Model file for the job. Use its own axes, mm. Round coordinates to 2 decimals unless told otherwise and drop trailing zeros. Loops run counter-clockwise (first coordinate to the right, second up) from the corner with the lowest first, then second, coordinate; pieces in that order, holes last. Notation, with made-up numbers: (-21.75, 2.5) -> (-12.75, 2.5) arc R19 cw to (-12.75, 7.5) -> close; hole circle Ø4 at (62, -35). An arc over 180 degrees is marked (long way). Use a Markdown table: item, result.
from build123d import *

# Parameters (mm, degrees)
CYLINDER041_R     = 1.5
CYLINDER041_DEPTH = 4
CYLINDER040_R     = 1.5
CYLINDER040_DEPTH = 4
CYLINDER042_R     = 1.5
CYLINDER042_DEPTH = 4
BOX010_W          = 1
BOX010_H          = 20
BOX010_DEPTH      = 1
BOX011_W          = 1
BOX011_H          = 20
BOX011_DEPTH      = 1
CYLINDER039_R     = 1.5
CYLINDER039_DEPTH = 4
BOX004_W          = 30
BOX004_H          = 73
BOX004_DEPTH      = 4
FILLET004_R       = 2


with BuildPart() as payload_plate_screw005:
    # Cylinder041 → Cylinder041 (new body)
    with BuildSketch(Plane(origin=(-10, 25, 152.7), x_dir=(1, 0, 0), z_dir=(0, 0, 1))):
        Circle(CYLINDER041_R)
    extrude(amount=CYLINDER041_DEPTH)


with BuildPart() as payload_plate_screw004:
    # Cylinder040 → Cylinder040 (new body)
    with BuildSketch(Plane(origin=(-10, -33, 152.7), x_dir=(1, 0, 0), z_dir=(0, 0, 1))):
        Circle(CYLINDER040_R)
    extrude(amount=CYLINDER040_DEPTH)


with BuildPart() as payload_plate_screw006:
    # Cylinder042 → Cylinder042 (new body)
    with BuildSketch(Plane(origin=(10, 25, 152.7), x_dir=(1, 0, 0), z_dir=(0, 0, 1))):
        Circle(CYLINDER042_R)
    extrude(amount=CYLINDER042_DEPTH)


with BuildPart() as center_plate001:
    # Box010 → Box010 (new body)
    with BuildSketch(Plane(origin=(-0.5, -10, 155.7), x_dir=(1, 0, 0), z_dir=(0, 0, 1))):
        with Locations((0.5, 10)):
            Rectangle(BOX010_W, BOX010_H)
    extrude(amount=BOX010_DEPTH)


with BuildPart() as payload_plate_center:
    # Box011 → Box011 (new body)
    with BuildSketch(Plane(origin=(10, -0.5, 155.7), x_dir=(0, 1, 0), z_dir=(0, 0, 1))):
        with Locations((0.5, 10)):
            Rectangle(BOX011_W, BOX011_H)
    extrude(amount=BOX011_DEPTH)

    # Fusion018: union center-plate001
    add(center_plate001.part)


with BuildPart() as payload_plate_screw_holes:
    # Cylinder039 → Cylinder039 (new body)
    with BuildSketch(Plane(origin=(10, -33, 152.7), x_dir=(1, 0, 0), z_dir=(0, 0, 1))):
        Circle(CYLINDER039_R)
    extrude(amount=CYLINDER039_DEPTH)

    # Compound003: union payload-plate-screw005, payload-plate-screw004, payload-plate-screw006, payload-plate-center
    add(payload_plate_screw005.part)
    add(payload_plate_screw004.part)
    add(payload_plate_screw006.part)
    add(payload_plate_center.part)


with BuildPart() as payload_plate:
    # Box004 → Box004 (new body)
    with BuildSketch(Plane(origin=(-15, -40.5, 152.7), x_dir=(1, 0, 0), z_dir=(0, 0, 1))):
        with Locations((15, 36.5)):
            Rectangle(BOX004_W, BOX004_H)
    extrude(amount=BOX004_DEPTH)

    # Fillet004
    fillet004_edges = [payload_plate.edges().sort_by_distance(p)[0] for p in [
        (0, -40.5, 156.7),
        (0, 32.5, 156.7),
    ]]
    fillet(fillet004_edges, radius=FILLET004_R)

    # Cut035: cut payload-plate-screw-holes
    add(payload_plate_screw_holes.part, mode=Mode.SUBTRACT)


solid = payload_plate.part
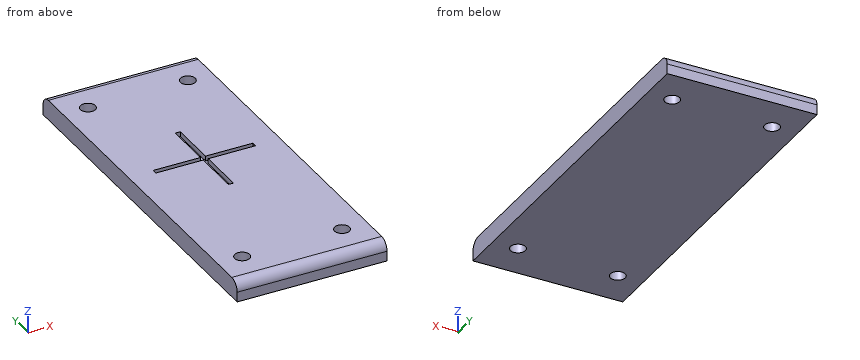
Q1. Band-saw the part on A-A, the plane y = 25. Give the cut face in (x, z), plus the area to 3 significant figures.
Results list:
| item | result |
|---|---|
| outline | (-15, 152.7) -> (-11.5, 152.7) -> (-11.5, 156.7) -> (-15, 156.7) -> close; (-8.5, 152.7) -> (8.5, 152.7) -> (8.5, 156.7) -> (-8.5, 156.7) -> close; (11.5, 152.7) -> (15, 152.7) -> (15, 156.7) -> (11.5, 156.7) -> close |
| area | 96.0 mm² |
Q2. Band-saw the part on B-B, the plane x = -9.25. Give the cut face in (y, z).
Results list:
| item | result |
|---|---|
| outline | (-40.5, 152.7) -> (-34.3, 152.7) -> (-34.3, 156.7) -> (-38.5, 156.7) arc R2 ccw to (-40.5, 154.7) -> close; (-31.7, 152.7) -> (23.7, 152.7) -> (23.7, 156.7) -> (0.5, 156.7) -> (0.5, 155.7) -> (-0.5, 155.7) -> (-0.5, 156.7) -> (-31.7, 156.7) -> close; (26.3, 152.7) -> (32.5, 152.7) -> (32.5, 154.7) arc R2 ccw to (30.5, 156.7) -> (26.3, 156.7) -> close |
Q3. Drill centre lines: L1, parallel to Y at x = -10, z = 154.45; L2, parallel to X at y = 8.5, z = 156.05; L3, parallel to Y at x = 9.5, z = 153.2. Where is each one in solid material? Low to high. Write a range as from..to.
Results list:
| item | result |
|---|---|
| L1 | y = -40.5..-34.5, -31.5..23.5, 26.5..32.5 |
| L2 | x = -15..-0.5, 0.5..15 |
| L3 | y = -40.5..-34.41, -31.59..23.59, 26.41..32.5 |
Q4. Flat gauge pins, fed straight in: pin 1 (0.5 mm diameter, centred on x = 4.5, z = 156, fed in from -Y); pin 2 (1.1 mm diameter, centred on x = 0, z = 156.5, fed in from -Y); pin 3 (1.8 mm diameter, centred on x = -10, y = 25, fed in from +Z); pin 4 (1.1 mm diameter, centred on x = 3.5, z = 156.5, fed in from +Y). Where does each tip first touch, or does it go through?
Results list:
| item | result |
|---|---|
| pin 1 | stops at y = -40.2 |
| pin 2 | stops at y = -40.06 |
| pin 3 | passes through |
| pin 4 | stops at y = 32.06 |
